Check sheet for the modelled part. Datum: model origin and axes. Units: mm. Give positions to 0.01 mm unless a question says otherwise; leave off trailing zeros. Order: outer loops, then holes, each group sorted by start corner. A loop starts at its lowest first (then second) coordinate and runs counter-clockwise, first axis right, second up.
Item 1: Sectioned sample at D-D on y = 127. Record the boundary of the cut face in (x, z), and give its area (3 significant figures).
Item 2: Release check for a two-part mould opening along Z. For faces 1 (the conical face through (1.6, 24.6, 23.5)), 2 (the flat face through (0, 29, 66)) record: released by +Z, released by -Z, zero draft, split by the parting line, or undercut.
Item 3: Sectioned sample at B-B on z = 46. Record the boundary of the cut face in (x, y), and give its area (3 significant figures).
Item 4: Material ranges on line 1 along Z through (x, y) = (1.9, 23.68); line 2 along Y through (x, z) = (1.8, 22); line 3 along Z through (x, y) = (0.8, 131.5), recorded low to high.
Item 5: Sectioned sample at C-C on x = 0.5. Count the separate pieces of the cut face and the enclosed holes in it, and give its area (3 significant figures).
Item 6: Sectioned sample at A-A on y = 43.5. Record the boundary of the cut face in (x, z), and give its area (3 significant figures).
Item 7: Gauge pin test, flat ends, axial feed: P1, Ø4.5, axis at y = 171, z = 22, coming from the -X side; P2, Ø3, axis at y = 23.68, z = 22, coming from the +X side. Record the tip position at first contact, or that the pin passes through.
from build123d import *

# Parameters (mm, degrees)
F0_W           = 180
F0_H           = 130
F1_DEPTH       = 2
F3_D           = 3.3
F3_CSINK_D     = 6.72
F3_CSINK_ANGLE = 90
F4_W           = 130
F4_H           = 95
F5_DEPTH       = 2.001
F7_D           = 4.4
F7_CSINK_D     = 8.96
F7_CSINK_ANGLE = 90


with BuildPart() as f1:
    # F0 (on Right) → F1 (new body)
    with BuildSketch(Plane.YZ):
        with Locations((90, 65)):
            Rectangle(F0_W, F0_H)
    extrude(amount=F1_DEPTH)

    # F3 (through all)
    with Locations(Plane(origin=(0, 0, 0), x_dir=(0, -1, 0), z_dir=(-1, 0, 0))):
        with Locations((-171, 108.36), (-171, 22), (-23.68, 22), (-23.68, 108.36)):
            CounterSinkHole(F3_D / 2, F3_CSINK_D / 2, counter_sink_angle=F3_CSINK_ANGLE)

    # F4 (on face) → F5 (cut, through all)
    with BuildSketch(Plane(origin=(0, 0, 0), x_dir=(0, -1, 0), z_dir=(-1, 0, 0))):
        with Locations((-98, 67.5)):
            Rectangle(F4_W, F4_H)
    extrude(amount=-F5_DEPTH, mode=Mode.SUBTRACT)

    # F7 (through all)
    with Locations(Plane(origin=(0, 0, 0), x_dir=(0, -1, 0), z_dir=(-1, 0, 0))):
        with Locations((-152.5, 7.5), (-43.5, 7.5), (-172.5, 122.5)):
            CounterSinkHole(F7_D / 2, F7_CSINK_D / 2, counter_sink_angle=F7_CSINK_ANGLE)


solid = f1.part
Report:
1. outline: (0, 0) - (2, 0) - (2, 20) - (0, 20) - close; (0, 115) - (2, 115) - (2, 130) - (0, 130) - close
1. area: 70.0 mm2
2. face 1: undercut
2. face 2: zero draft
3. outline: (0, 0) - (2, 0) - (2, 33) - (0, 33) - close; (0, 163) - (2, 163) - (2, 180) - (0, 180) - close
3. area: 100 mm2
4. line 1: z = 0 to 20.35, 23.65 to 106.71, 110.01 to 130
4. line 2: y = 0 to 22.03, 25.33 to 33, 163 to 169.35, 172.65 to 180
4. line 3: z = 0 to 20, 115 to 130
5. separate pieces: 1
5. enclosed holes: 8
5. area: 10,800 mm2
6. outline: (0, 0) - (2, 0) - (2, 5.02) - (0, 3.02) - close; (0, 11.98) - (2, 9.98) - (2, 20) - (0, 20) - close; (0, 115) - (2, 115) - (2, 130) - (0, 130) - close
6. area: 56.1 mm2
7. P1: stops at x = 1.11
7. P2: passes through
